Read the model definition and answer for the solid it produces. Units are mm, in the model's axes. A direction names the side the tool comes from. Give positions to 0.01 mm unless a question says otherwise; leave off trailing zeros. Write each loop counter-clockwise with the first axis right and the second up, starting at its lowest first coordinate (ties: lowest second). Pieces come first, ordered by that corner, then holes.
```python
from build123d import *

# Parameters (mm, degrees)
SKETCH_R        = 10.25
PAD_DEPTH       = 25
SKETCH001_R     = 1.75
POCKET_DEPTH    = 22.501
POCKET001_DEPTH = 3
CHAMFER_SIZE2   = 12
CHAMFER_SIZE    = 3
FILLET_R        = 3
FILLET001_R     = 3


with BuildPart() as part:
    # Sketch → Pad (new body)
    with BuildSketch(Plane.XY):
        with BuildLine():
            ThreePointArc((15, 0), (3.882286, 14.488887), (-12.990381, 7.5))
            Line((-12.990381, 7.5), (-26.990381, 7.5))
            Line((-26.990381, 7.5), (-26.990381, 2.5))
            Line((-26.990381, 2.5), (-14.990381, 2.5))
            Line((-14.990381, 2.5), (-14.990381, -2.5))
            Line((-26.990381, -2.5), (-14.990381, -2.5))
            Line((-26.990381, -7.5), (-26.990381, -2.5))
            Line((-12.990381, -7.5), (-26.990381, -7.5))
            ThreePointArc((-12.990381, -7.5), (3.882286, -14.488887), (15, 0))
        make_face()
        Circle(SKETCH_R, mode=Mode.SUBTRACT)
    extrude(amount=PAD_DEPTH)

    # Sketch001 (on Face8 of Pad) → Pocket (cut, through all)
    with BuildSketch(Plane.XZ.offset(7.5)):
        with Locations((-20, 6)):
            Circle(SKETCH001_R)
        with Locations((-20, 18)):
            Circle(SKETCH001_R)
    extrude(amount=-POCKET_DEPTH, mode=Mode.SUBTRACT)

    # Sketch002 (on Face3 of Pocket) → Pocket001 (cut)
    with BuildSketch(Plane(origin=(0, 7.5, 0), x_dir=(-1, 0, 0), z_dir=(0, 1, 0))):
        Polygon((20, 2.75), (22.814583, 4.375), (22.814583, 7.625), (20, 9.25), (17.185417, 7.625), (17.185417, 4.375), align=None)
        Polygon((20, 14.75), (22.814583, 16.375), (22.814583, 19.625), (20, 21.25), (17.185417, 19.625), (17.185417, 16.375), align=None)
    extrude(amount=-POCKET001_DEPTH, mode=Mode.SUBTRACT)

    # Chamfer
    chamfer_edges = [part.edges().sort_by_distance(p)[0] for p in [
        (-26.990381, 5, 0),
        (-26.990381, -5, 0),
    ]]
    chamfer_side = part.faces().sort_by_distance((3.748719, 13.990411, 0))[0]
    chamfer(chamfer_edges, length=CHAMFER_SIZE, length2=CHAMFER_SIZE2, reference=chamfer_side)

    # Fillet
    fillet_edges = [part.edges().sort_by_distance(p)[0] for p in [
        (-23.990381, 5, 0),
        (-23.990381, -5, 0),
    ]]
    fillet(fillet_edges, radius=FILLET_R)

    # Fillet001
    fillet001_edges = [part.edges().sort_by_distance(p)[0] for p in [
        (3.882286, -14.488887, 0),
        (3.882286, 14.488887, 0),
    ]]
    fillet(fillet001_edges, radius=FILLET001_R)


solid = part.part
```
Item 1: Determine the mould class of faces 1 (the flat face through (-18.573, 6.021, 3.574)), 2 (the flat face through (-11, 0, 0)), 3 (the flat face through (-26.99, 5, 18)) for opening direction X: pulls with the +X half, pulls with the -X half, needs draft (parallel to the pull), parting line crosses it, or undercut.
Result set:
face 1: undercut
face 2: needs draft
face 3: pulls with the -X half
Item 2: Find the intervals of material crossed by line 1 along Z through (x, y) = (-20, -4.2); line 2 along Y through (x, z) = (0, 7); line 3 along X through (y, z) = (-5, 19.25), in increasing order.
Result set:
line 1: z = 0 to 4.25, 7.75 to 16.25, 19.75 to 25
line 2: y = -15 to -10.25, 10.25 to 15
line 3: x = -26.99 to -21.22, -18.78 to -8.95, 8.95 to 14.14
Item 3: Section C-C (z = 11) is taken. Write down the section's boundary in (x, y).
Result set:
outline: (-26.74, -7.5) - (-12.99, -7.5) arc R15 ccw (long way) to (-12.99, 7.5) - (-26.74, 7.5) - (-26.74, 2.5) - (-14.99, 2.5) - (-14.99, -2.5) - (-26.74, -2.5) - close; hole circle Ø20.5 at (0, 0)
Item 4: Section D-D (z = 6) is taken. Write down the section's boundary in (x, y), and give its area (3 significant figures).
Result set:
outline: (-25.49, -7.5) - (-21.75, -7.5) - (-21.75, -2.5) - (-25.49, -2.5) - close; (-25.49, 2.5) - (-21.75, 2.5) - (-21.75, 4.5) - (-22.81, 4.5) - (-22.81, 7.5) - (-25.49, 7.5) - close; (-18.25, -7.5) - (-12.99, -7.5) arc R15 ccw (long way) to (-12.99, 7.5) - (-17.19, 7.5) - (-17.19, 4.5) - (-18.25, 4.5) - (-18.25, 2.5) - (-14.99, 2.5) - (-14.99, -2.5) - (-18.25, -2.5) - close; hole circle Ø20.5 at (0, 0)
area: 450 mm2
Item 5: Section A-A (z = 18) is taken. Write down the section's boundary in (x, y).
Result set:
outline: (-26.99, -7.5) - (-21.75, -7.5) - (-21.75, -2.5) - (-26.99, -2.5) - close; (-26.99, 2.5) - (-21.75, 2.5) - (-21.75, 4.5) - (-22.81, 4.5) - (-22.81, 7.5) - (-26.99, 7.5) - close; (-18.25, -7.5) - (-12.99, -7.5) arc R15 ccw (long way) to (-12.99, 7.5) - (-17.19, 7.5) - (-17.19, 4.5) - (-18.25, 4.5) - (-18.25, 2.5) - (-14.99, 2.5) - (-14.99, -2.5) - (-18.25, -2.5) - close; hole circle Ø20.5 at (0, 0)
Item 6: Each of these flat-tipped pins is pushed along its axis until it touches: pin 1 Ø14 at (x, z) = (-16, 16) entering from +Y; pin 2 Ø6 at (x, z) = (-21.5, 16) entering from +Y; pin 3 Ø2.5 at (y, z) = (6, 6.5) entering from -X. Where does it stop, or does it pass through?
Result set:
pin 1: stops at y = 12
pin 2: stops at y = 7.5
pin 3: stops at x = -25.93
Item 7: Which of the six approach directions +Z, -Z, +X, -X, +Y, -Y give full straight-line access (tool end or side, diameter ignored) to faces 4 (the flat face through (-18.612, 6.021, 20.449)), 5 (the flat face through (-21, -2.5, 12)), 6 (the cylindrical face through (-21.39, 3.49, 4.94))?
Result set:
face 4: +Y
face 5: +Z, -Z, -X
face 6: +Y, -Y
Item 8: Section B-B (x = -21) is taken. Give the number of separate pieces and of enclosed holes in the cut face, and give its area (3 significant figures).
Result set:
separate pieces: 6
enclosed holes: 0
area: 178 mm2
